from build123d import *

# Parameters (mm, degrees)
SKETCH1_W            = 110
SKETCH1_H            = 130
BOSS_EXTRUDE1_DEPTH  = 5
SKETCH10_W           = 110
SKETCH10_H           = 60
BOSS_EXTRUDE4_DEPTH  = 13
SKETCH6_R            = 21
CUT_EXTRUDE2_DEPTH   = 30
BOSS_EXTRUDE8_DEPTH  = 50
SKETCH23_R           = 13
CUT_EXTRUDE5_DEPTH   = 130.464280788
SKETCH26_R           = 2
CUT_EXTRUDE8_DEPTH   = 10
CUT_EXTRUDE23_START  = -50
CUT_EXTRUDE23_DEPTH  = 50
SKETCH37_R           = 1.5
CUT_EXTRUDE25_DEPTH  = 4
BOSS_EXTRUDE10_START = 2
SKETCH39_W           = 110
SKETCH39_H           = 130
SKETCH39_R           = 21
SKETCH39_R_2         = 1.5
BOSS_EXTRUDE10_DEPTH = 2
SKETCH41_W           = 50
SKETCH41_H           = 29.177777778
CUT_EXTRUDE26_DEPTH  = 7
SKETCH43_R           = 2
CUT_EXTRUDE27_DEPTH  = 9


with BuildPart() as part:
    # Sketch1 → Boss-Extrude1 (new, symmetric)
    with BuildSketch(Plane.XY):
        with Locations((0, 5)):
            Rectangle(SKETCH1_W, SKETCH1_H)
    extrude(amount=BOSS_EXTRUDE1_DEPTH, both=True)

    # Sketch10 → Boss-Extrude4 (add)
    with BuildSketch(Plane.XZ.offset(60)):
        with Locations((0, 25)):
            Rectangle(SKETCH10_W, SKETCH10_H)
    extrude(amount=-BOSS_EXTRUDE4_DEPTH)

    # Sketch6 → Cut-Extrude2 (cut)
    with BuildSketch(Plane(origin=(0, 0, -5), x_dir=(-1, 0, 0), z_dir=(0, 0, -1))):
        with Locations((0, 20)):
            Circle(SKETCH6_R)
    extrude(amount=-CUT_EXTRUDE2_DEPTH, mode=Mode.SUBTRACT)

    # Sketch18 → Boss-Extrude8 (add)
    with BuildSketch(Plane.XY.offset(5)):
        with BuildLine():
            Line((-55, -47), (-39, -47))
            Line((-39, -47), (-39, -17.822222222))
            Line((-39, -17.822222222), (-30.482216757, -17.822222222))
            Line((-30.482216757, -17.822222222), (-30.482216757, -14.450463881))
            ThreePointArc((-30.482216757, -14.450463881), (0, 66), (30.482216757, -14.450463881))
            Line((30.482216757, -14.450463881), (30.482216757, -17.822222222))
            Line((30.482216757, -17.822222222), (39, -17.822222222))
            Line((39, -17.822222222), (39, -47))
            Line((39, -47), (55, -47))
            Line((55, -47), (55, 70))
            Line((55, 70), (-55, 70))
            Line((-55, 70), (-55, -47))
        make_face()
    extrude(amount=BOSS_EXTRUDE8_DEPTH)

    # Sketch23 → Cut-Extrude5 (cut, through all)
    with BuildSketch(Plane(origin=(-39, 0, 0), x_dir=(0, 0, -1), z_dir=(1, 0, 0))):
        with Locations((-25, -32)):
            Circle(SKETCH23_R)
    cut_extrude5 = extrude(amount=-CUT_EXTRUDE5_DEPTH, mode=Mode.SUBTRACT)

    # Sketch26 → Cut-Extrude8 (cut)
    with BuildSketch(Plane.XY.offset(55)):
        with Locations((-45, 60)):
            Circle(SKETCH26_R)
        with Locations(Location((45, 60, 0), (0, 0, 180))):
            Circle(SKETCH26_R)
        with Locations((-47, -52)):
            Circle(SKETCH26_R)
        with Locations(Location((47, -52, 0), (0, 0, 180))):
            Circle(SKETCH26_R)
        with Locations((-45, -12)):
            Circle(SKETCH26_R)
        with Locations((45, -12)):
            Circle(SKETCH26_R)
    extrude(amount=-CUT_EXTRUDE8_DEPTH, mode=Mode.SUBTRACT)

    # Sketch31 → Cut-Extrude23 (cut)
    with BuildSketch(Plane.XY.offset(55).offset(CUT_EXTRUDE23_START)):
        with BuildLine():
            Line((-9.539392014, 65), (-45, 65))
            ThreePointArc((-45, 65), (-41.464466094, 63.535533906), (-40, 60))
            ThreePointArc((-40, 60), (-45, 55), (-50, 60))
            Line((-50, 60), (-50, -2.822222222))
            Line((-50, -2.822222222), (-39.939281076, -2.822222222))
            ThreePointArc((-39.939281076, -2.822222222), (-41.976162634, 38.814934773), (-9.539392014, 65))
        make_face()
        with BuildLine():
            Line((9.539392014, 65), (-9.539392014, 65))
            ThreePointArc((-9.539392014, 65), (-41.976162634, 38.814934773), (-39.939281076, -2.822222222))
            Line((-39.939281076, -2.822222222), (39.939281076, -2.822222222))
            ThreePointArc((39.939281076, -2.822222222), (41.976162634, 38.814934773), (9.539392014, 65))
        make_face()
        with BuildLine():
            Line((45, 65), (9.539392014, 65))
            ThreePointArc((9.539392014, 65), (41.976162634, 38.814934773), (39.939281076, -2.822222222))
            Line((39.939281076, -2.822222222), (50, -2.822222222))
            Line((50, -2.822222222), (50, 60))
            ThreePointArc((50, 60), (41.464466094, 56.464466094), (45, 65))
        make_face()
    extrude(amount=CUT_EXTRUDE23_DEPTH, mode=Mode.SUBTRACT)

    # Sketch37 → Cut-Extrude25 (cut)
    with BuildSketch(Plane(origin=(0, 0, -5), x_dir=(-1, 0, 0), z_dir=(0, 0, -1))):
        with Locations((-17, 37)):
            Circle(SKETCH37_R)
        with Locations(Location((17, 37, 0), (0, 0, 180))):
            Circle(SKETCH37_R)
        with Locations(Location((-17, 3, 0), (0, 0, 180))):
            Circle(SKETCH37_R)
        with Locations((17, 3)):
            Circle(SKETCH37_R)
    extrude(amount=-CUT_EXTRUDE25_DEPTH, mode=Mode.SUBTRACT)

    # Sketch39 → Boss-Extrude10 (add)
    with BuildSketch(Plane(origin=(0, 0, -5), x_dir=(-1, 0, 0), z_dir=(0, 0, -1)).offset(BOSS_EXTRUDE10_START)):
        with Locations((0, 5)):
            Rectangle(SKETCH39_W, SKETCH39_H)
        with Locations((0, 20)):
            Circle(SKETCH39_R, mode=Mode.SUBTRACT)
        with Locations((-17, 37)):
            Circle(SKETCH39_R_2, mode=Mode.SUBTRACT)
        with Locations((17, 37)):
            Circle(SKETCH39_R_2, mode=Mode.SUBTRACT)
        with Locations((17, 3)):
            Circle(SKETCH39_R_2, mode=Mode.SUBTRACT)
        with Locations((-17, 3)):
            Circle(SKETCH39_R_2, mode=Mode.SUBTRACT)
    extrude(amount=-BOSS_EXTRUDE10_DEPTH)

    # Sketch41 → Cut-Extrude26 (cut)
    with BuildSketch(Plane(origin=(-39, 0, 0), x_dir=(0, 0, -1), z_dir=(1, 0, 0))):
        with Locations((-30, -32.411111111)):
            Rectangle(SKETCH41_W, SKETCH41_H)
    cut_extrude26 = extrude(amount=-CUT_EXTRUDE26_DEPTH, mode=Mode.SUBTRACT)

    # Mirror1: Cut-Extrude26 across plane
    add(cut_extrude26.mirror(Plane(origin=(0, 0, 0), x_dir=(0, 0, 1), z_dir=(1, 0, 0))), mode=Mode.SUBTRACT)

    # Mirror2: Cut-Extrude5 across plane
    add(cut_extrude5.mirror(Plane(origin=(0, 0, 0), x_dir=(0, 0, 1), z_dir=(1, 0, 0))), mode=Mode.SUBTRACT)

    # Sketch43 → Cut-Extrude27 (cut)
    with BuildSketch(Plane(origin=(55, 0, 0), x_dir=(0, 0, -1), z_dir=(1, 0, 0))):
        with Locations((-25, -11)):
            Circle(SKETCH43_R)
        with Locations((-4, -32)):
            Circle(SKETCH43_R)
        with Locations((-25, -53)):
            Circle(SKETCH43_R)
        with Locations((-46, -32)):
            Circle(SKETCH43_R)
    cut_extrude27 = extrude(amount=-CUT_EXTRUDE27_DEPTH, mode=Mode.SUBTRACT)

    # Mirror3: Cut-Extrude27 across plane
    add(cut_extrude27.mirror(Plane(origin=(0, 0, 0), x_dir=(0, 0, 1), z_dir=(1, 0, 0))), mode=Mode.SUBTRACT)


solid = part.part
The model under review builds one solid part; all positions refer to its coordinate system, in mm. A direction names the side the tool comes from. Round coordinates to 2 decimals unless told otherwise and drop trailing zeros. Write each loop counter-clockwise with the first axis right and the second up, starting at its lowest first coordinate (ties: lowest second). Pieces come first, ordered by that corner, then holes. Notation, with made-up numbers: (64.25, -21) - (106.25, -21) arc R28 ccw to (106.25, 7) - close; hole circle Ø3 at (44.5, 32.25). An arc over 180 degrees is marked (long way). One line per item, written item: value. Start each with the question number.
1. Consider section B-B on x = 25. Write out the cut boundary in (y, z), and give its area (3 significant figures).
2. To check wall thickness, follow L1, parallel to X at y = 58.5, z = 24; L2, parallel to X at y = 37, z = 19.5; L3, parallel to Y at x = -51.25, z = 25. State the ranges of each line that lie inside material, in increasing order. Write a range as from..to.
3. The part is to be moulded in two halves that separate along X. For faces 1 (the face through (1, -60, 24)), 2 (the face through (50, 28, 30)), 3 (the face through (46, -32, 4)), say which applies: released by +X, released by -X, zero draft, split by the parting line, or undercut.
4. Consider section A-A on y = -32. State how many separate pieces and enclosed holes the cut face has, and give its area (3 significant figures).
5. Consider section C-C on y = 15. Write out the cut boundary in (x, z).
6. Clearance check with flat-ended pins moving along their axes: P1, Ø6, axis at x = -16.5, y = -24.5, coming from the +Z side; P2, Ø1.5, axis at x = 17, y = 3.5, coming from the -Z side; P3, Ø3.5, axis at y = -32, z = 46, coming from the -X side; P4, Ø2.5, axis at y = -32, z = 4, coming from the +X side. State where each tip first meets the part, or that it passes through.
7. Machinability: for faces 4 (the face through (17, 37, -1)), 5 (the face through (-45, -2.822, 30)), 6 (the face through (50.6, -54.2, 26.6)), which of the approach directions +Z, -Z, +X, -X, +Y, -Y give a long, thin tool a straight path to every point of the face, cutting with its end or side? Answer none if there is none.
Checks:
1. outline: (-60, -7) - (70, -7) - (70, 55) - (65, 55) - (65, 5) - (-47, 5) - (-47, 55) - (-60, 55) - close
1. area: 2,460 mm^2
2. L1: x = -55..-50, -49.77..-40.23, 40.23..49.77, 50..55
2. L2: x = -55..-50, 50..55
2. L3: y = -60..-55, -51..-45, -19..-13, -9..70
3. face 1: zero draft
3. face 2: undercut
3. face 3: released by +X
4. separate pieces: 7
4. enclosed holes: 0
4. area: 1,610 mm^2
5. outline: (-55, -7) - (-20.4, -7) - (-20.4, 5) - (-50, 5) - (-50, 55) - (-55, 55) - close; (20.4, -7) - (55, -7) - (55, 55) - (50, 55) - (50, 5) - (20.4, 5) - close
6. P1: stops at z = 5
6. P2: stops at z = -1
6. P3: passes through
6. P4: stops at x = 46
7. face 4: -Z
7. face 5: +Z
7. face 6: +X
